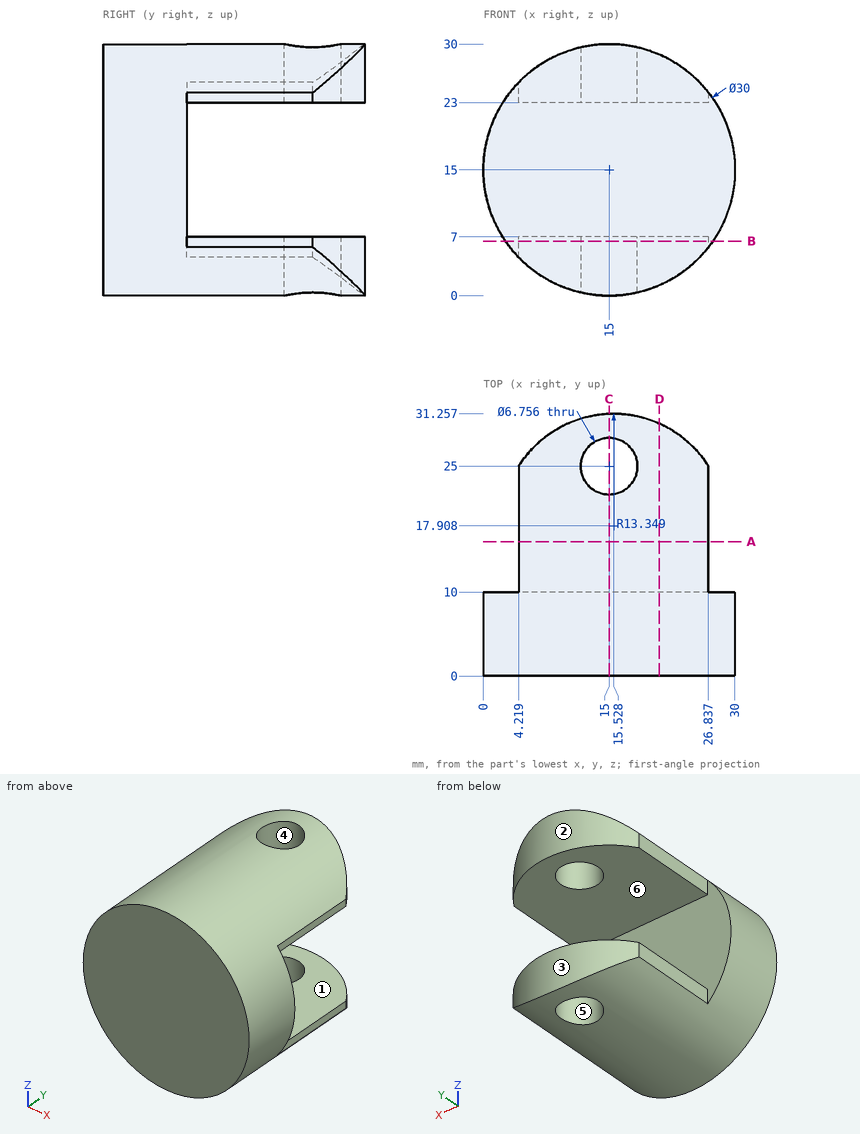
Could you check a few things on this drawing? It's one solid part, dimensions in mm from its lowest x, y, z. A direction names the side the tool comes from. Give positions to 0.01 mm unless a question says otherwise; leave off trailing zeros. Order: outer loops, then holes, each group sorted by start corner. A loop starts at its lowest first (then second) coordinate and runs counter-clockwise, first axis right, second up. Notation, with made-up numbers: (4.5, -24.5) -> (37.5, -24.5) arc R26 ccw to (37.5, 1.5) -> close; hole circle Ø5 at (29.25, -26). An arc over 180 degrees is marked (long way). Use CSV: the item, a comma, the result in double quotes. Start each with the question number.
Item 1: If I drill on probe 1 along Y at (x, z) = (15, 1.5); probe 2 along Y at (x, z) = (12.5, 12); probe 3 along Z at (x, y) = (20, 16), over which ranges is the centre line in solid material (lowest first)? Write a range as [from, to].
Item 2: Suppose I cut it at D-D (x = 21). List the corners of the cut face in (y, z) for me.
Item 3: Suppose I cut it at C-C (x = 15). List the corners of the cut face in (y, z) for me, and give its area (3 significant figures).
Item 4: Suppose I cut it at B-B (z = 6.5). List the corners of the cut face in (x, y) for me.
Item 5: I'm going to push flat-ended pins straight in: P1, Ø0.6, axis at y = 17, z = 23.5, coming from the +X side; P2, Ø1.5, axis at x = 10.5, z = 17.5, coming from the +Y side; P3, Ø0.7, axis at y = 19, z = 23.5, coming from the -X side. Where does each tip first touch, or does it pass through?
Item 6: Thinking about a two-plate mould opening in X: for the marked faces 3, 4, 5 and 6, which applies, pulls with the +X half, pulls with the -X half, needs draft (parallel to the pull), parting line crosses it, or undercut?
Item 7: Suppose I cut it at A-A (y = 16). List the corners of the cut face in (x, z) for me.
Item 8: On a 3-axis mill with a long thin cutter (end or side, diameter ignored), from which of +Z, -Z, +X, -X, +Y, -Y can I reach the whole of each face in a straight line? I mean the marked faces 1 and 2. Say none if no direction works.
Answer block:
1,probe 1,"y = [0, 21.62], [28.38, 31.25]"
1,probe 2,"y = [0, 10]"
1,probe 3,"z = [0.86, 7], [23, 29.14]"
2,outline,"(0, 1.25) -> (30.08, 1.25) -> (30.08, 7) -> (10, 7) -> (10, 23) -> (30.08, 23) -> (30.08, 28.75) -> (0, 28.75) -> close"
3,outline,"(0, 0) -> (21.62, 0) -> (21.62, 7) -> (10, 7) -> (10, 23) -> (21.62, 23) -> (21.62, 30) -> (0, 30) -> close; (28.38, 0) -> (31.25, 0) -> (31.25, 7) -> (28.38, 7) -> close; (28.38, 23) -> (31.25, 23) -> (31.25, 30) -> (28.38, 30) -> close"
3,area,"503 mm^2"
4,outline,"(2.64, 0) -> (27.36, 0) -> (27.36, 10) -> (26.84, 10) -> (26.84, 25) arc R13.35 ccw to (4.22, 25) -> (4.22, 10) -> (2.64, 10) -> close; hole circle Ø6.76 at (15, 25)"
5,P1,"stops at x = 26.84"
5,P2,"stops at y = 10"
5,P3,"stops at x = 4.22"
6,face 3,"parting line crosses it"
6,face 4,"undercut"
6,face 5,"undercut"
6,face 6,"needs draft"
7,outline,"(4.22, 4.57) arc R15 ccw to (26.84, 5.79) -> (26.84, 7) -> (4.22, 7) -> close; (4.22, 23) -> (26.84, 23) -> (26.84, 24.21) arc R15 ccw to (4.22, 25.43) -> close"
8,face 1,"+X, -X, +Y"
8,face 2,"+Z, -Z, +Y"
